Can you work these out from the model? Positions are in its coordinate system, mm. A direction names the side the tool comes from. Coordinates: 2 decimals unless noted, no trailing zeros. Order: outer loops, then holes, each group sorted by start corner. A loop starts at its lowest first (then second) coordinate and runs counter-clockwise, first axis right, second up. Notation, with made-up numbers: (47.5, -32.75) -> (100.5, -32.75) arc R22 cw to (100.5, -2.75) -> close; hole circle Ø9 at (21.5, -5.5). An arc over 180 degrees is marked (long way). Answer as a JSON object with one key per item and string values. Group by question number.
(1) I want a section at C-C, the plane x = 7.5. State how many separate pieces and enclosed holes the cut face has, plus the area to 3 significant figures.
(2) For pin 1 (2.5 mm diameter, centred on x = 20, z = -132.5, fed in from +Y); pin 2 (13 mm diameter, centred on y = 18, z = -31, fed in from +X); pin 3 (9 mm diameter, centred on x = 12.5, z = -14, fed in from +Y), each with a flat end and sliding along its axis, tell me the tip position at first contact or that it passes through.
(3) Which directions (+Z, -Z, +X, -X, +Y, -Y) give clear straight access to the entire face, cutting with the end or side of a thin tool? Please do faces 4 (the flat face through (15, 2, 0)), 5 (the flat face through (15, 57.7, -130)), 6 (the flat face through (15, 59, -59)).
(4) I need wall thicknesses on line 1 (X direction, y = 1.15, z = -7.5); line 2 (Z direction, x = 26.75, y = 22.5); line 3 (Y direction, x = 17.75, z = -51). Which ranges of each line are inside material? Lowest first, please.
(5) I want a section at B-B, the plane z = -7.5. List the corners of the cut face in (x, y) for me, plus the area to 3 significant figures.
(6) If we mould it in two halves opening along Y, with no side actions, what happens to faces 1 (the flat face through (15, 57.7, -50)), 2 (the flat face through (15, 64, -50)), 3 (the flat face through (16.5, 11, -34))? For each: pulls with the +Y half, pulls with the -Y half, needs draft (parallel to the pull), parting line crosses it, or undercut.
(7) I want a section at D-D, the plane y = 20. List the corners of the cut face in (x, z) for me, plus the area to 3 significant figures.
(8) I want a section at A-A, the plane y = 38. List the corners of the cut face in (x, z) for me.
from build123d import *

# Parameters (mm, degrees)
SKETCH1_W           = 30
SKETCH1_H           = 45
BOSS_EXTRUDE1_DEPTH = 4
SKETCH2_W           = 30
SKETCH2_H           = 4
BOSS_EXTRUDE2_DEPTH = 58
SKETCH7_W           = 3
SKETCH7_H           = 41
BOSS_EXTRUDE3_DEPTH = 41
CUT_EXTRUDE1_DEPTH  = 3
SKETCH10_R          = 2
CUT_EXTRUDE2_DEPTH  = 4
CHAMFER1_SIZE       = 1
BOSS_EXTRUDE4_DEPTH = 15
SKETCH12_W          = 3.5
SKETCH12_H          = 3
CUT_EXTRUDE3_DEPTH  = 30
SKETCH13_W          = 18
SKETCH13_H          = 2
BOSS_EXTRUDE5_DEPTH = 30
SKETCH14_W          = 1
SKETCH14_H          = 54
CUT_EXTRUDE4_DEPTH  = 30
SKETCH15_W          = 3.75
SKETCH15_H          = 0.3
BOSS_EXTRUDE6_DEPTH = 30
FILLET1_R           = 3


with BuildPart() as part:
    # Sketch1 → Boss-Extrude1 (new body)
    with BuildSketch(Plane(origin=(0, 0, 0), x_dir=(1, 0, 0), z_dir=(0, 1, 0))):
        with Locations((15, 22.5)):
            Rectangle(SKETCH1_W, SKETCH1_H)
    extrude(amount=BOSS_EXTRUDE1_DEPTH)

    # Sketch2 → Boss-Extrude2 (add)
    with BuildSketch(Plane(origin=(0, 4, 0), x_dir=(1, 0, 0), z_dir=(0, 1, 0))):
        with Locations((15, 43)):
            Rectangle(SKETCH2_W, SKETCH2_H)
    extrude(amount=BOSS_EXTRUDE2_DEPTH)

    # Sketch7 → Boss-Extrude3 (add)
    with BuildSketch(Plane(origin=(0, 4, 0), x_dir=(1, 0, 0), z_dir=(0, 1, 0))):
        with Locations((15, 20.5)):
            Rectangle(SKETCH7_W, SKETCH7_H)
    extrude(amount=BOSS_EXTRUDE3_DEPTH)

    # Sketch8 → Cut-Extrude1 (cut)
    with BuildSketch(Plane(origin=(16.5, 0, 0), x_dir=(0, 0, -1), z_dir=(1, 0, 0))):
        Polygon((41, 45), (0, 45), (0, 4), (15, 4), (41, 30), align=None)
    extrude(amount=-CUT_EXTRUDE1_DEPTH, mode=Mode.SUBTRACT)

    # Sketch10 → Cut-Extrude2 (cut)
    with BuildSketch(Plane(origin=(0, 4, 0), x_dir=(1, 0, 0), z_dir=(0, 1, 0))):
        with Locations(Location((7.5, 7.5, 0), (0, 0, 270))):
            Circle(SKETCH10_R)
        with Locations(Location((22.5, 7.5, 0), (0, 0, 270))):
            Circle(SKETCH10_R)
        with Locations(Location((22.5, 33.5, 0), (0, 0, 90))):
            Circle(SKETCH10_R)
        with Locations(Location((7.5, 33.5, 0), (0, 0, 90))):
            Circle(SKETCH10_R)
    extrude(amount=-CUT_EXTRUDE2_DEPTH, mode=Mode.SUBTRACT)

    # Chamfer1
    chamfer1_edges = [part.edges().sort_by_distance(p)[0] for p in [
        (7.5, 4, -31.5),
        (22.5, 4, -31.5),
        (22.5, 4, -9.5),
        (7.5, 4, -9.5),
    ]]
    chamfer(chamfer1_edges, length=CHAMFER1_SIZE)

    # Sketch11 → Boss-Extrude4 (add, symmetric)
    with BuildSketch(Plane(origin=(15, 0, 0), x_dir=(0, 0, -1), z_dir=(1, 0, 0))):
        Polygon((45, 0), (137, 0), (137, 62), (128, 62), (128, 58), (133, 58), (133, 4), (49, 4), (49, 58), (59, 58), (59, 62), (45, 62), align=None)
    extrude(amount=BOSS_EXTRUDE4_DEPTH, both=True)

    # Sketch12 → Cut-Extrude3 (cut)
    with BuildSketch(Plane.ZY):
        with Locations((-53.5, 59.5)):
            Rectangle(SKETCH12_W, SKETCH12_H)
    extrude(amount=-CUT_EXTRUDE3_DEPTH, mode=Mode.SUBTRACT)

    # Sketch13 → Boss-Extrude5 (add)
    with BuildSketch(Plane(origin=(30, 0, 0), x_dir=(0, 0, -1), z_dir=(1, 0, 0))):
        with Locations((50, 63)):
            Rectangle(SKETCH13_W, SKETCH13_H)
    extrude(amount=-BOSS_EXTRUDE5_DEPTH)

    # Sketch14 → Cut-Extrude4 (cut)
    with BuildSketch(Plane.ZY):
        with Locations((-48.5, 31)):
            Rectangle(SKETCH14_W, SKETCH14_H)
    extrude(amount=-CUT_EXTRUDE4_DEPTH, mode=Mode.SUBTRACT)

    # Sketch15 → Boss-Extrude6 (add)
    with BuildSketch(Plane.ZY):
        with Locations((-57.125, 57.85)):
            Rectangle(SKETCH15_W, SKETCH15_H)
        Polygon((-51.75, 58), (-51.75, 57.7), (-48.3, 57.7), (-48.3, 4.3), (-132.7, 4.3), (-132.7, 57.7), (-128, 57.7), (-128, 58), (-133, 58), (-133, 4), (-48, 4), (-48, 58), align=None)
    extrude(amount=-BOSS_EXTRUDE6_DEPTH)

    # Fillet1
    fillet1_edges = [part.edges().sort_by_distance(p)[0] for p in [
        (15, 64, -41),
        (15, 64, -59),
        (15, 62, -128),
        (15, 62, -137),
    ]]
    fillet(fillet1_edges, radius=FILLET1_R)


solid = part.part
Computed values:
{
 "1": {"separate pieces": "3", "enclosed holes": "0", "area": "1,300 mm2"},
 "2": {"pin 1": "stops at y = 62", "pin 2": "stops at x = 16.5", "pin 3": "stops at y = 7.39"},
 "3": {"face 4": "+Z, +X, -X, +Y, -Y", "face 5": "+X, -X", "face 6": "+X, -X, +Y"},
 "4": {"line 1": "x = 0 to 5.5, 9.5 to 20.5, 24.5 to 30", "line 2": "z = -137 to -132.7, -48.3 to -41", "line 3": "y = 0 to 4.3, 57.7 to 64"},
 "5": {"outline": "(0, 0) -> (5.5, 0) -> (5.5, 3) -> (4.5, 4) -> (0, 4) -> close; (9.5, 0) -> (20.5, 0) -> (20.5, 3) -> (19.5, 4) -> (10.5, 4) -> (9.5, 3) -> close; (24.5, 0) -> (30, 0) -> (30, 4) -> (25.5, 4) -> (24.5, 3) -> close", "area": "86.0 mm2"},
 "6": {"face 1": "undercut", "face 2": "pulls with the +Y half", "face 3": "needs draft"},
 "7": {"outline": "(0, -137) -> (30, -137) -> (30, -132.7) -> (0, -132.7) -> close; (0, -48.3) -> (30, -48.3) -> (30, -41) -> (16.5, -41) -> (16.5, -31) -> (13.5, -31) -> (13.5, -41) -> (0, -41) -> close", "area": "378 mm2"},
 "8": {"outline": "(0, -137) -> (30, -137) -> (30, -132.7) -> (0, -132.7) -> close; (0, -48.3) -> (30, -48.3) -> (30, -41) -> (0, -41) -> close"}
}
